Check sheet for the modelled part. Datum: model origin and axes. Units: mm. Round coordinates to 2 decimals unless told otherwise and drop trailing zeros. Write each loop counter-clockwise with the first axis right and the second up, starting at its lowest first coordinate (ties: lowest second). Pieces come first, ordered by that corner, then holes. Notation, with made-up numbers: (83, 81.25) -> (138, 81.25) arc R12 cw to (138, 96.25) -> close; hole circle Ø6 at (64.5, 8.5). An arc over 180 degrees is marked (long way). One line per item, written item: value.
from build123d import *

# Parameters (mm, degrees)
SKETCH002_R      = 2
SKETCH002_R_2    = 1.5
EXTRUDE001_DEPTH = 4


with BuildPart() as part:
    # Sketch002 → Extrude001 (new body)
    with BuildSketch(Plane.XY):
        with BuildLine():
            Line((-8, -92.933243), (-8, -17.000938))
            ThreePointArc((-8, -17.000938), (-8.297069, -14.84111), (-9.166214, -12.841687))
            ThreePointArc((3.732527, 23.29894), (-11.329683, 8.302585), (-9.166214, -12.841687))
            ThreePointArc((6.882805, 18.381245), (7.254673, 22.087346), (3.732527, 23.29894))
            ThreePointArc((6.882805, 18.381245), (6.118525, 16.652055), (6.660919, 14.84097))
            ThreePointArc((8.798632, -11.457288), (11.535462, 2.001195), (6.660919, 14.84097))
            ThreePointArc((8.798632, -11.457288), (8.20259, -13.032404), (8, -14.704293))
            Line((8, -14.704293), (8, -45.025379))
            Line((8, -45.025379), (8, -92.933243))
            Line((0, -100.933243), (8, -92.933243))
            Line((-8, -92.933243), (0, -100.933243))
        make_face()
        with Locations((0, -75)):
            Circle(SKETCH002_R, mode=Mode.SUBTRACT)
        with Locations((0, -93.433243)):
            Circle(SKETCH002_R_2, mode=Mode.SUBTRACT)
        with Locations((6.717514, 6.717514)):
            Circle(SKETCH002_R_2, mode=Mode.SUBTRACT)
        with Locations((5.656854, -5.656854)):
            Circle(SKETCH002_R_2, mode=Mode.SUBTRACT)
        with Locations((-6.717514, -6.717514)):
            Circle(SKETCH002_R_2, mode=Mode.SUBTRACT)
        with Locations((-5.656854, 5.656854)):
            Circle(SKETCH002_R_2, mode=Mode.SUBTRACT)
    extrude(amount=-EXTRUDE001_DEPTH)


solid = part.part
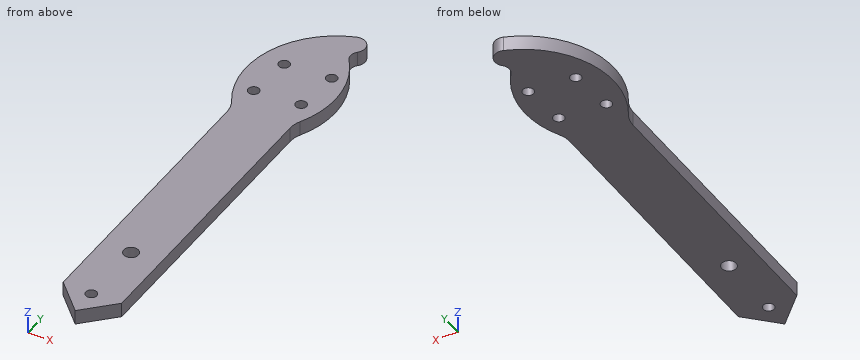
Item 1: Depth check by flat-ended pin: P1, Ø1.2, axis at y = -62, z = -3, coming from the -X side; P2, Ø5, axis at x = 0, y = -75, coming from the +Z side; P3, Ø2, axis at x = -1.5, z = -3.5, coming from the +Y side; P4, Ø2, axis at y = -61, z = -1.5, coming from the +X side. Enter the tip coordinate at first touch or a pass-through.
Answer:
P1: stops at x = -8
P2: stops at z = 0
P3: stops at y = 21.34
P4: stops at x = 8
Item 2: Thickness scan on line 1 (Y direction, x = 5.75, z = -3.1); line 2 (Y direction, x = 6.75, z = -1.1); line 3 (Y direction, x = 0.25, z = -1.4). Record the ranges inside material, lowest first.
Answer:
line 1: y = -95.18 to -7.15, -4.16 to 5.57, 7.86 to 23.29
line 2: y = -94.18 to -6.68, -4.63 to 5.22, 8.22 to 14.72, 18.23 to 22.69
line 3: y = -100.68 to -94.91, -91.95 to -76.98, -73.02 to 21.76
Item 3: Sectioned sample at C-C on y = -21. Enter the section's corners in (x, z).
Answer:
outline: (-8, -4) -> (8, -4) -> (8, 0) -> (-8, 0) -> close
Item 4: Sectioned sample at B-B on z = -2. Enter the section's corners in (x, y), and give its area (3 significant figures).
Answer:
outline: (-9.17, -12.84) arc R8 cw to (-8, -17) -> (-8, -92.93) -> (0, -100.93) -> (8, -92.93) -> (8, -14.7) arc R7 cw to (8.8, -11.46) arc R24.7 ccw to (6.66, 14.84) arc R2.73 cw to (6.88, 18.38) arc R3 ccw to (3.73, 23.3) arc R24.7 ccw to start; hole circle Ø3 at (-6.72, -6.72); hole circle Ø3 at (-5.66, 5.66); hole circle Ø4 at (0, -75); hole circle Ø3 at (0, -93.43); hole circle Ø3 at (5.66, -5.66); hole circle Ø3 at (6.72, 6.72)
area: 1,980 mm^2
Item 5: Sectioned sample at A-A on y = -75. Enter the section's corners in (x, z).
Answer:
outline: (-8, -4) -> (-2, -4) -> (-2, 0) -> (-8, 0) -> close; (2, -4) -> (8, -4) -> (8, 0) -> (2, 0) -> close
